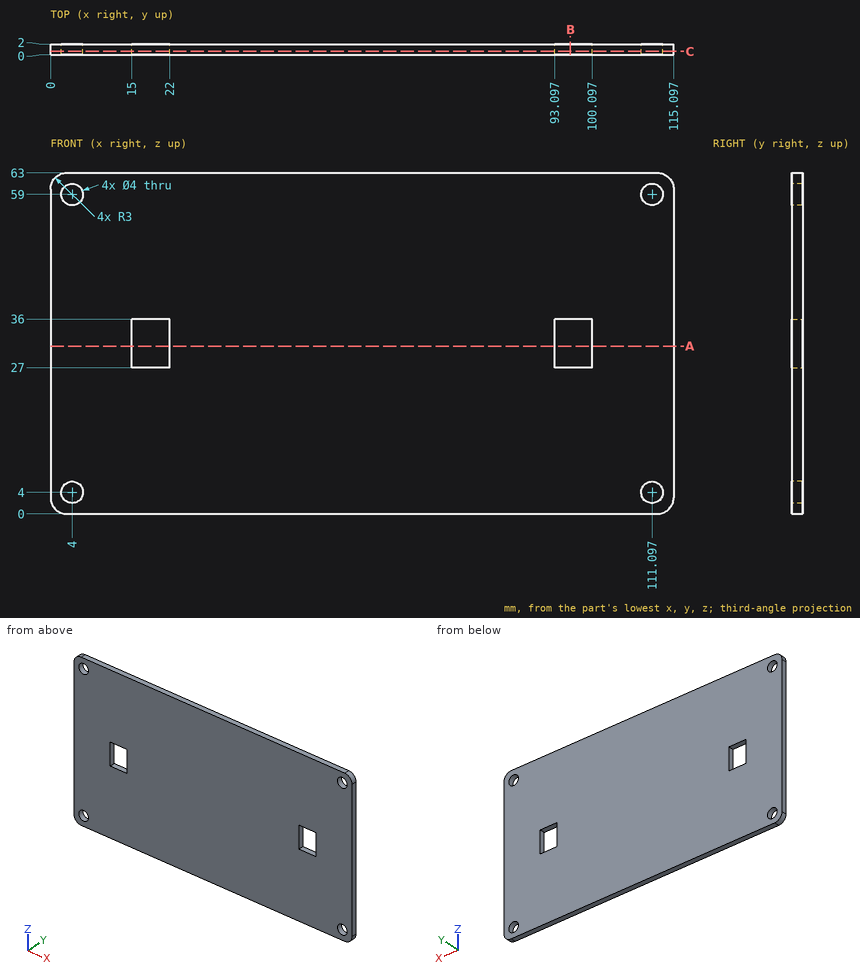
Design review of the part shown in the three views and the two pictorial views. Dimensions are in mm from the part's minimum x, y and z. Coordinates: 2 decimals unless noted, no trailing zeros. Order: outer loops, then holes, each group sorted by start corner. A loop starts at its lowest first (then second) coordinate and runs counter-clockwise, first axis right, second up. Notation, with made-up numbers: (-39, 63.5) - (-31, 63.5) arc R6 cw to (-31, 73.5) - close; hole circle Ø3 at (4.5, 33.5). An arc over 180 degrees is marked (long way). One line per question, with ' | ' between items.
Q1. Clearance check with a flat-ended pin moving along its axis: pin 1 Ø5 at (x, z) = (111.1, 4) entering from -Y. State where the tip first meets the part, or that it passes through.
Answer key:
pin 1: stops at y = 0
Q2. Consider section B-B, the plane x = 96. Give the boundary of the cut face in (y, z), then the cut area to 3 significant figures.
Answer key:
outline: (0, 0) - (2, 0) - (2, 27) - (0, 27) - close; (0, 36) - (2, 36) - (2, 63) - (0, 63) - close | area: 108 mm2
Q3. Consider section A-A, the plane z = 31. Give the boundary of the cut face in (x, y).
Answer key:
outline: (0, 0) - (15, 0) - (15, 2) - (0, 2) - close; (22, 0) - (93.1, 0) - (93.1, 2) - (22, 2) - close; (100.1, 0) - (115.1, 0) - (115.1, 2) - (100.1, 2) - close
Q4. Consider section C-C, the plane y = 0.65. Give the boundary of the cut face in (x, z), then the cut area to 3 significant figures.
Answer key:
outline: (0, 3) arc R3 ccw to (3, 0) - (112.1, 0) arc R3 ccw to (115.1, 3) - (115.1, 60) arc R3 ccw to (112.1, 63) - (3, 63) arc R3 ccw to (0, 60) - close; hole circle Ø4 at (4, 4); hole circle Ø4 at (4, 59); hole (15, 27) - (22, 27) - (22, 36) - (15, 36) - close; hole (93.1, 27) - (100.1, 27) - (100.1, 36) - (93.1, 36) - close; hole circle Ø4 at (111.1, 4); hole circle Ø4 at (111.1, 59) | area: 7,070 mm2
Q5. To check wall thickness, follow line 1 along X through (y, z) = (1.2, 4); line 2 along X through (y, z) = (0.2, 34); line 3 along Z through (x, y) = (95.5, 1.2). State the ranges of each line that lie inside material, in increasing order.
Answer key:
line 1: x = 0 to 2, 6 to 109.1, 113.1 to 115.1 | line 2: x = 0 to 15, 22 to 93.1, 100.1 to 115.1 | line 3: z = 0 to 27, 36 to 63
